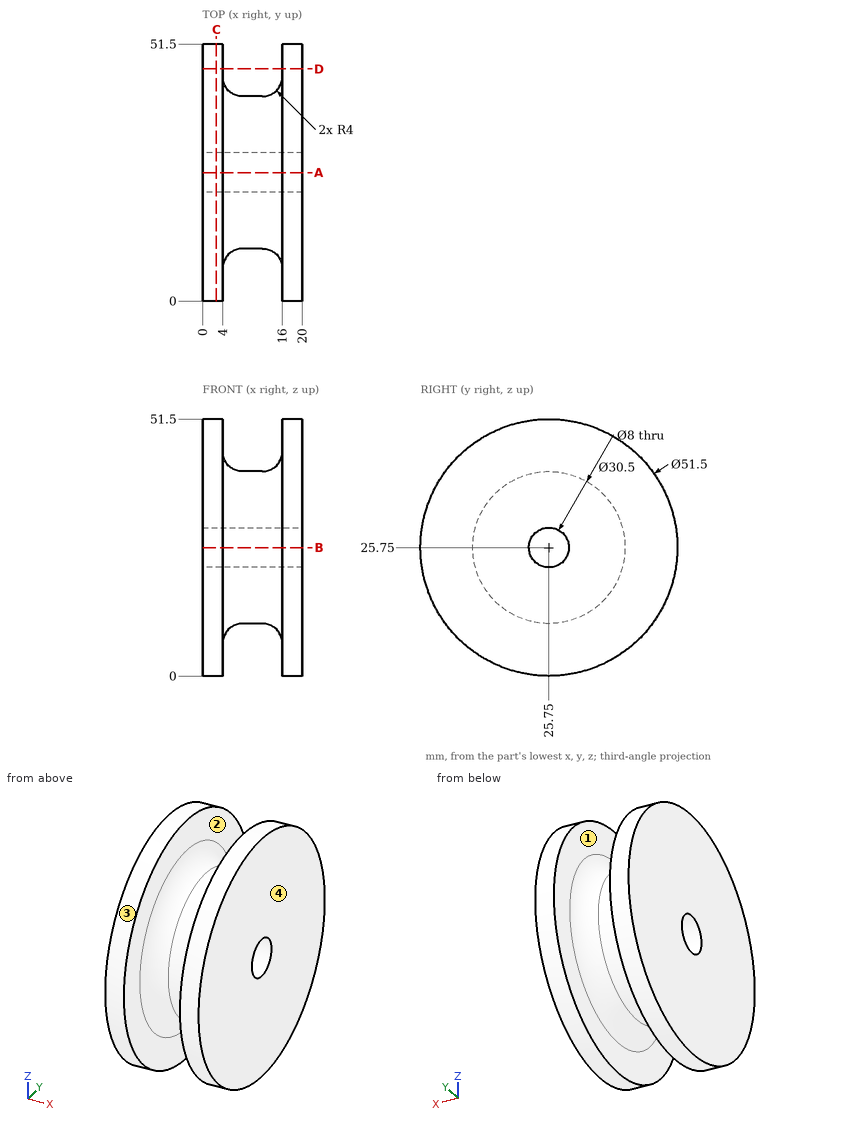
Design review of the part shown in the three views and the two pictorial views. Dimensions are in mm from the part's minimum x, y and z. Round coordinates to 2 decimals unless told otherwise and drop trailing zeros. Order: outer loops, then holes, each group sorted by start corner. A loop starts at its lowest first (then second) coordinate and runs counter-clockwise, first axis right, second up.
Item 1: Draft analysis for pull direction X (two halves, no side actions). For the marked faces 1, 2, 3 and 4, state which applies: released by +X, released by -X, zero draft, split by the parting line, or undercut.
Working result:
face 1: undercut
face 2: undercut
face 3: zero draft
face 4: released by +X
Item 2: To check wall thickness, follow probe 1 along X at (y, z) = (5.5, 31); probe 2 along Y at (x, z) = (11, 25.75); probe 3 along Z at (x, y) = (11, 26.5). State the ranges of each line that lie inside material, in increasing order.
Working result:
probe 1: x = 0 to 4, 16 to 20
probe 2: y = 10.5 to 21.75, 29.75 to 41
probe 3: z = 10.52 to 21.82, 29.68 to 40.98
Item 3: Add section A-A, the plane y = 25.75. State the section outline as (x, z) points.
Working result:
outline: (0, 0) - (4, 0) - (4, 6.5) arc R4 cw to (8, 10.5) - (12, 10.5) arc R4 cw to (16, 6.5) - (16, 0) - (20, 0) - (20, 21.75) - (0, 21.75) - close; (0, 29.75) - (20, 29.75) - (20, 51.5) - (16, 51.5) - (16, 45) arc R4 cw to (12, 41) - (8, 41) arc R4 cw to (4, 45) - (4, 51.5) - (0, 51.5) - close
Item 4: Add section D-D, the plane y = 46.5. State the section outline as (x, z) points.
Working result:
outline: (0, 10.5) - (4, 10.5) - (4, 41) - (0, 41) - close; (16, 10.5) - (20, 10.5) - (20, 41) - (16, 41) - close
Item 5: For pin 1 (1.5 mm diameter, centred on x = 12.5, y = 19, fed in from +Z); pin 2 (1 mm diameter, centred on x = 5.5, z = 16, fed in from -Y); pin 3 (3 mm diameter, centred on x = 8, y = 39, fed in from -Z); pin 4 (6.5 mm diameter, centred on y = 25.75, z = 25.75, fed in from -X), all flat-tipped, find the tip position at first contact; note any pin that passes through.
Working result:
pin 1: stops at z = 39.83
pin 2: stops at y = 12.22
pin 3: stops at z = 16.03
pin 4: passes through
Item 6: Add section C-C, the plane x = 2.75. State the section outline as (y, z) points.
Working result:
outline: circle Ø51.5 at (25.75, 25.75); hole circle Ø8 at (25.75, 25.75)
